from build123d import *

# Parameters (mm, degrees)
SKETCH1_W           = 40
SKETCH1_H           = 50
SKETCH1_R           = 2
BOSS_EXTRUDE1_DEPTH = 8
BOSS_EXTRUDE2_DEPTH = 25


with BuildPart() as part:
    # Sketch1 → Boss-Extrude1 (new body)
    with BuildSketch(Plane(origin=(0, 0, 0), x_dir=(1, 0, 0), z_dir=(0, 1, 0))):
        Rectangle(SKETCH1_W, SKETCH1_H)
        with Locations(Location((-10, -17, 0), (0, 0, 270))):
            Circle(SKETCH1_R, mode=Mode.SUBTRACT)
        with Locations(Location((10, -17, 0), (0, 0, 90))):
            Circle(SKETCH1_R, mode=Mode.SUBTRACT)
    extrude(amount=BOSS_EXTRUDE1_DEPTH)

    # Sketch2 → Boss-Extrude2 (add)
    with BuildSketch(Plane(origin=(0, 8, 0), x_dir=(1, 0, 0), z_dir=(0, 1, 0))):
        Polygon((-4, 25), (4, 25), (4, 15), (14, 15), (14, 7), (4, 7), (4, -3), (-4, -3), (-4, 7), (-14, 7), (-14, 15), (-4, 15), align=None)
    extrude(amount=BOSS_EXTRUDE2_DEPTH)


solid = part.part
Could you check a few things on this model? Use its own coordinates, in mm. A direction names the side the tool comes from. Give positions to 0.01 mm unless a question says otherwise; leave off trailing zeros. Write each loop counter-clockwise with the first axis right and the second up, starting at its lowest first coordinate (ties: lowest second). Pieces come first, ordered by that corner, then holes. Notation, with made-up numbers: (13.5, 44.5) -> (20.5, 44.5) arc R15 ccw to (20.5, 52.5) -> close; hole circle Ø11 at (36.25, -5.5). An arc over 180 degrees is marked (long way). Answer as a JSON object with one key per item and string values.
Q1. We'd pull the mould along Z, two halves only. Please class faces 5 (the cylindrical face through (-8.648, 3.944, 15.526)), 6 (the flat face through (-2, 10, -25)), 7 (the flat face through (0, 4, 25)), 8 (the flat face through (0, 33, -11)): released by +Z, released by -Z, zero draft, split by the parting line, or undercut.
Taken from the geometry:
{"face 5": "undercut", "face 6": "released by -Z", "face 7": "released by +Z", "face 8": "zero draft"}
Q2. Suppose I cut it at C-C on y = 29.5. Write out the boundary of the cut face in (x, z), then the cut area to 3 significant figures.
Taken from the geometry:
{"outline": "(-14, -15) -> (-4, -15) -> (-4, -25) -> (4, -25) -> (4, -15) -> (14, -15) -> (14, -7) -> (4, -7) -> (4, 3) -> (-4, 3) -> (-4, -7) -> (-14, -7) -> close", "area": "384 mm²"}
Q3. Suppose I cut it at D-D on z = 12. Write out the boundary of the cut face in (x, y), then the cut area to 3 significant figures.
Taken from the geometry:
{"outline": "(-20, 0) -> (20, 0) -> (20, 8) -> (-20, 8) -> close", "area": "320 mm²"}
Q4. Which directions (+Z, -Z, +X, -X, +Y, -Y) give clear straight access to the entire face, cutting with the end or side of a thin tool? Please do faces 1 (the flat face through (9, 20, -7)), 2 (the flat face through (-4, 20, -20)), 3 (the flat face through (-9, 20, -7)), 4 (the flat face through (4, 20, -20)).
Taken from the geometry:
{"face 1": "+Z, +X, +Y", "face 2": "-Z, -X, +Y", "face 3": "+Z, -X, +Y", "face 4": "-Z, +X, +Y"}
Q5. Will these pins go through, and if not, where does the flat tip stop? pin 1 Ø1.5 at (x, z) = (7.5, 6.5) entering from +Y; pin 2 Ø11 at (y, z) = (17.5, -18.5) entering from -X; pin 3 Ø8 at (y, z) = (19, -17.5) entering from +X; pin 4 Ø3.5 at (x, z) = (10, 17) entering from -Y.
Taken from the geometry:
{"pin 1": "stops at y = 8", "pin 2": "stops at x = -14", "pin 3": "stops at x = 14", "pin 4": "passes through"}
Q6. Suppose I cut it at B-B on x = 10. Write out the boundary of the cut face in (y, z), then the cut area to 3 significant figures.
Taken from the geometry:
{"outline": "(0, -25) -> (8, -25) -> (8, -15) -> (33, -15) -> (33, -7) -> (8, -7) -> (8, 15) -> (0, 15) -> close; (0, 19) -> (8, 19) -> (8, 25) -> (0, 25) -> close", "area": "568 mm²"}
Q7. Suppose I cut it at A-A on z = 17. Write out the boundary of the cut face in (x, y), then the cut area to 3 significant figures.
Taken from the geometry:
{"outline": "(-20, 0) -> (-12, 0) -> (-12, 8) -> (-20, 8) -> close; (-8, 0) -> (8, 0) -> (8, 8) -> (-8, 8) -> close; (12, 0) -> (20, 0) -> (20, 8) -> (12, 8) -> close", "area": "256 mm²"}
Q8. Please list where these lines run through material, in increasing order: L1, parallel to X at y = 3, z = 17; L2, parallel to Z at x = 10, y = 3; L3, parallel to X at y = 15, z = -17.
Taken from the geometry:
{"L1": "x = -20 to -12, -8 to 8, 12 to 20", "L2": "z = -25 to 15, 19 to 25", "L3": "x = -4 to 4"}
